Work out the finished part from the listing and answer in its coordinate system (mm). Face numbers are marked on the shaded views. A direction names the side the tool comes from. Give positions to 0.01 mm unless a question says otherwise; leave off trailing zeros. Order: outer loops, then holes, each group sorted by start corner. A loop starts at its lowest first (then second) coordinate and runs counter-clockwise, first axis right, second up. Notation, with made-up numbers: M 73.5,-34.75 L 122.5,-34.75 A26 ccw 122.5,-10.75 Z; hole C 35.5,-31.75 d4. An arc over 180 degrees is marked long. One line per item, written item: value.
from build123d import *

# Parameters (mm, degrees)
SKETCH1_R           = 15
BOSS_EXTRUDE1_DEPTH = 5
SKETCH2_R           = 5
BOSS_EXTRUDE2_DEPTH = 90
CUT_EXTRUDE1_START  = -15
CUT_EXTRUDE1_DEPTH  = 15
SKETCH4_W           = 2
SKETCH4_H           = 5.2
CUT_EXTRUDE2_DEPTH  = 99.17076958
FILLET1_R           = 10
FILLET2_R           = 2
CUT_EXTRUDE3_DEPTH  = 1
SKETCH6_R           = 13.5
SKETCH6_R_2         = 11.5
CUT_EXTRUDE4_DEPTH  = 1


with BuildPart() as part:
    # Sketch1 → Boss-Extrude1 (new body)
    with BuildSketch(Plane(origin=(0, 0, 0), x_dir=(1, 0, 0), z_dir=(0, 1, 0))):
        with Locations(Location((0, 0, 0), (0, 0, 270))):
            Circle(SKETCH1_R)
    extrude(amount=BOSS_EXTRUDE1_DEPTH)

    # Sketch2 → Boss-Extrude2 (add)
    with BuildSketch(Plane(origin=(0, 5, 0), x_dir=(1, 0, 0), z_dir=(0, 1, 0))):
        with Locations(Location((0, 0, 0), (0, 0, 90))):
            Circle(SKETCH2_R)
    extrude(amount=BOSS_EXTRUDE2_DEPTH)

    # Sketch3 → Cut-Extrude1 (cut)
    with BuildSketch(Plane(origin=(0, 95, 0), x_dir=(1, 0, 0), z_dir=(0, 1, 0)).offset(CUT_EXTRUDE1_START)):
        with BuildLine():
            Line((0, 5), (5, 0))
            ThreePointArc((5, 0), (3.535533906, 3.535533906), (0, 5))
        make_face()
    extrude(amount=CUT_EXTRUDE1_DEPTH, mode=Mode.SUBTRACT)

    # Sketch4 → Cut-Extrude2 (cut, through all)
    with BuildSketch(Plane(origin=(2.5, 0, -2.5), x_dir=(-0.7071067811865475, 0, -0.7071067811865477), z_dir=(0.7071067811865477, 0, -0.7071067811865475))):
        with Locations((0, 87.5)):
            Rectangle(SKETCH4_W, SKETCH4_H)
    extrude(amount=-CUT_EXTRUDE2_DEPTH, mode=Mode.SUBTRACT)

    # Fillet1
    fillet1_edges = [part.edges().sort_by_distance(p)[0] for p in [
        (0, 5, 5),
    ]]
    fillet(fillet1_edges, radius=FILLET1_R - 0.0001)  # a hair under: the kernel refuses the full size

    # Fillet2
    fillet2_edges = [part.edges().sort_by_distance(p)[0] for p in [
        (0, 5, -15),
    ]]
    fillet(fillet2_edges, radius=FILLET2_R)

    # Sketch5 → Cut-Extrude3 (cut)
    with BuildSketch(Plane.XZ):
        Polygon((-5.546534945, 7.181387117), (4.296413773, -2.661561601), (7.972695825, 1.01472045), (9.290003517, -0.302587242), (0.443849671, -9.148741088), (-0.873458021, -7.831433396), (2.818849671, -4.139125704), (-7.024099047, 5.703823014), align=None)
    extrude(amount=-CUT_EXTRUDE3_DEPTH, mode=Mode.SUBTRACT)

    # Sketch6 → Cut-Extrude4 (cut)
    with BuildSketch(Plane.XZ):
        with Locations(Location((0, 0, 0), (0, 0, 270))):
            Circle(SKETCH6_R)
        with Locations(Location((0, 0, 0), (0, 0, 270))):
            Circle(SKETCH6_R_2, mode=Mode.SUBTRACT)
    extrude(amount=-CUT_EXTRUDE4_DEPTH, mode=Mode.SUBTRACT)


solid = part.part
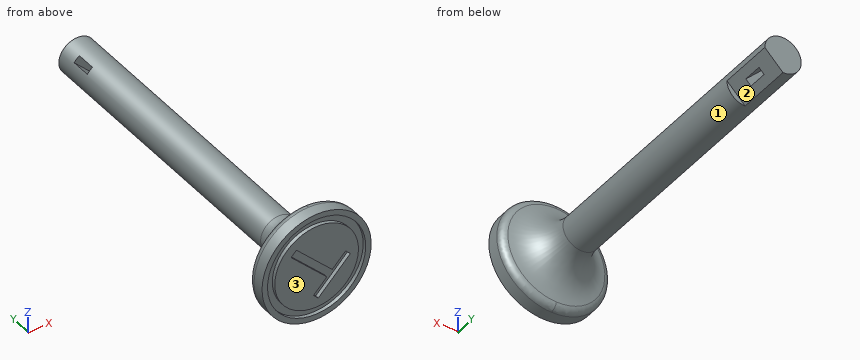
(1) Section A-A, the plane y = 13.5 is taken. Give the vertices of the cut face in (x, z), then the cut area to 3 significant figures.
Findings:
outline: C 0,0 d10.23
area: 82.1 mm^2
(2) Given P1, Ø8, axis at x = 4.5, z = -7.5, coming from the +Y side; P2, Ø5, axis at x = 9, y = 84, coming from the +Z side; P3, Ø6, axis at x = 1, z = 0.5, coming from the -Y side; P4, Ø6, axis at x = -1.5, z = 9.5, coming from the +Y side, each flat-ended and moving along its own axis, determine where each tip first touches the part or whether it passes through.
Findings:
P1: stops at y = 80
P2: passes through
P3: stops at y = 0
P4: stops at y = 9.55
(3) Which of the six approach directions +Z, -Z, +X, -X, +Y, -Y give full straight-line access (tool end or side, diameter ignored) to the marked faces 1, 2 and 3?
Findings:
face 1: +Y
face 2: -Z, +X, +Y
face 3: +Z, -Z, +X, -X, -Y
(4) Find the intervals of material crossed by probe 1 along X at (y, z) = (0.3, 0); probe 2 along Y at (x, z) = (9.5, -10); probe 3 along Z at (x, y) = (0, 81.5), in increasing order. Write a range as from..to.
Findings:
probe 1: x = -15..-13.5, -11.5..-1.32, 1.63..6.96, 8.99..11.5, 13.5..15
probe 2: y = 0..5
probe 3: z = -5..5
(5) Section B-B, the plane y = 42 is taken. Give the vertices of the cut face in (x, z).
Findings:
outline: C 0,0 d10
